Read the model definition and answer for the solid it produces. Units are mm, in the model's axes. Round coordinates to 2 decimals unless told otherwise and drop trailing zeros. Write each loop counter-clockwise with the first axis right and the second up, starting at its lowest first coordinate (ties: lowest second). Pieces come first, ordered by that corner, then holes. Notation, with made-up numbers: (50.25, -5) - (104.25, -5) arc R17 ccw to (104.25, 5) - close; hole circle Ø8 at (64, 70). An arc over 180 degrees is marked (long way). Answer as CSV lines item,"result". Start each with the question number.
1) Find section B-B on x = 52. Determine the outline of the cut face in (y, z).
2) Find section A-A on z = 41.5. Determine the outline of the cut face in (x, y), then the cut area to 3 significant figures.
3) Each of these flat-tipped pins is pushed along its axis until it touches: pin 1 (2 mm diameter, centred on x = -46.5, y = 1.5, fed in from -Z); pin 2 (1.5 mm diameter, centred on x = -6, y = 1.5, fed in from +Z); pin 3 (3.5 mm diameter, centred on x = -50.61, z = 49.27, fed in from -Y); pin 4 (5 mm diameter, centred on x = 1, z = -32.5, fed in from -Y). Where does it stop, or does it pass through?
4) Consider line 1 along X through (y, z) = (0.9, 49); line 2 along X through (y, z) = (1.6, 14.5); line 3 along X through (y, z) = (4.35, -22). Determine where each line is inside the solid, lowest interval first.
5) Find section C-C on y = 1.35. Determine the outline of the cut face in (x, z).
6) Find section D-D on x = 26.5. Determine the outline of the cut face in (y, z), then the cut area to 3 significant figures.
from build123d import *

# Parameters (mm, degrees)
SKETCH1_R           = 2.25
BOSS_EXTRUDE1_DEPTH = 5
CUT_EXTRUDE1_DEPTH  = 5


with BuildPart() as part:
    # Sketch1 → Boss-Extrude1 (new body)
    with BuildSketch(Plane(origin=(0, 0, 0), x_dir=(1, 0, 0), z_dir=(0, 1, 0))):
        Polygon((0, 55.733260811), (0, 12.733260811), (-65.613421019, 12.733260811), (-65.613421019, -54.266739189), (67.386578981, -54.266739189), (67.386578981, 55.733260811), align=None)
        with Locations((62.386578981, 40.733260811)):
            Circle(SKETCH1_R, mode=Mode.SUBTRACT)
        with Locations((62.386578981, 15.733260811)):
            Circle(SKETCH1_R, mode=Mode.SUBTRACT)
        with Locations((62.386578981, -9.266739189)):
            Circle(SKETCH1_R, mode=Mode.SUBTRACT)
        with Locations((62.386578981, -34.266739189)):
            Circle(SKETCH1_R, mode=Mode.SUBTRACT)
        with Locations((0.886578981, -49.266739189)):
            Circle(SKETCH1_R, mode=Mode.SUBTRACT)
        with Locations((-50.613421019, -49.266739189)):
            Circle(SKETCH1_R, mode=Mode.SUBTRACT)
        with Locations((52.386578981, -49.266739189)):
            Circle(SKETCH1_R, mode=Mode.SUBTRACT)
    extrude(amount=BOSS_EXTRUDE1_DEPTH)

    # Sketch2 → Cut-Extrude1 (cut)
    with BuildSketch(Plane(origin=(0, 5, 0), x_dir=(1, 0, 0), z_dir=(0, 1, 0))):
        Polygon((-8, -3), (42, -3), (42, -54.266739189), (-8, -54.266739189), (-31, -54.266739189), (-31, -3), align=None)
    extrude(amount=-CUT_EXTRUDE1_DEPTH, mode=Mode.SUBTRACT)


solid = part.part
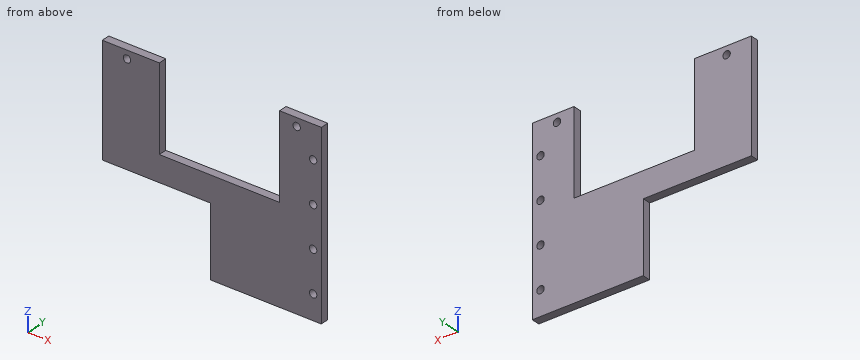
Check values:
1,outline,"(0, -55.73) - (5, -55.73) - (5, 47.05) - (0, 47.05) - close; (0, 51.48) - (5, 51.48) - (5, 54.27) - (0, 54.27) - close"
2,outline,"(-65.61, 0) - (-31, 0) - (-31, 5) - (-65.61, 5) - close; (42, 0) - (67.39, 0) - (67.39, 5) - (42, 5) - close"
2,area,"300 mm^2"
3,pin 1,"stops at z = -12.73"
3,pin 2,"stops at z = 3"
3,pin 3,"passes through"
3,pin 4,"stops at y = 0"
4,line 1,"x = -65.61 to -52.85, -48.38 to -31, 42 to 50.15, 54.62 to 67.39"
4,line 2,"x = -65.61 to -31, 42 to 67.39"
4,line 3,"x = 0 to 67.39"
5,outline,"(-65.61, -12.73) - (0, -12.73) - (0, -55.73) - (67.39, -55.73) - (67.39, 54.27) - (42, 54.27) - (42, 3) - (-31, 3) - (-31, 54.27) - (-65.61, 54.27) - close; hole circle Ø4.5 at (-50.61, 49.27); hole circle Ø4.5 at (52.39, 49.27); hole circle Ø4.5 at (62.39, -40.73); hole circle Ø4.5 at (62.39, -15.73); hole circle Ø4.5 at (62.39, 9.27); hole circle Ø4.5 at (62.39, 34.27)"
6,outline,"(0, -55.73) - (5, -55.73) - (5, 3) - (0, 3) - close"
6,area,"294 mm^2"
